Geometry: see drawing. Coordinates: mm, zero at the bounding-box minimum. A direction names the side the tool comes from. Round coordinates to 2 decimals unless told otherwise and drop trailing zeros. Loops run counter-clockwise (first coordinate to the right, second up) from the corner with the lowest first, then second, coordinate; pieces in that order, holes last. Notation, with made-up numbers: M -0.5,24 L 46.5,24 A16 ccw 46.5,47 Z; hole C 80.5,15.25 d2. An arc over 180 degrees is marked long. Answer as a JSON object with one key per item and string values.
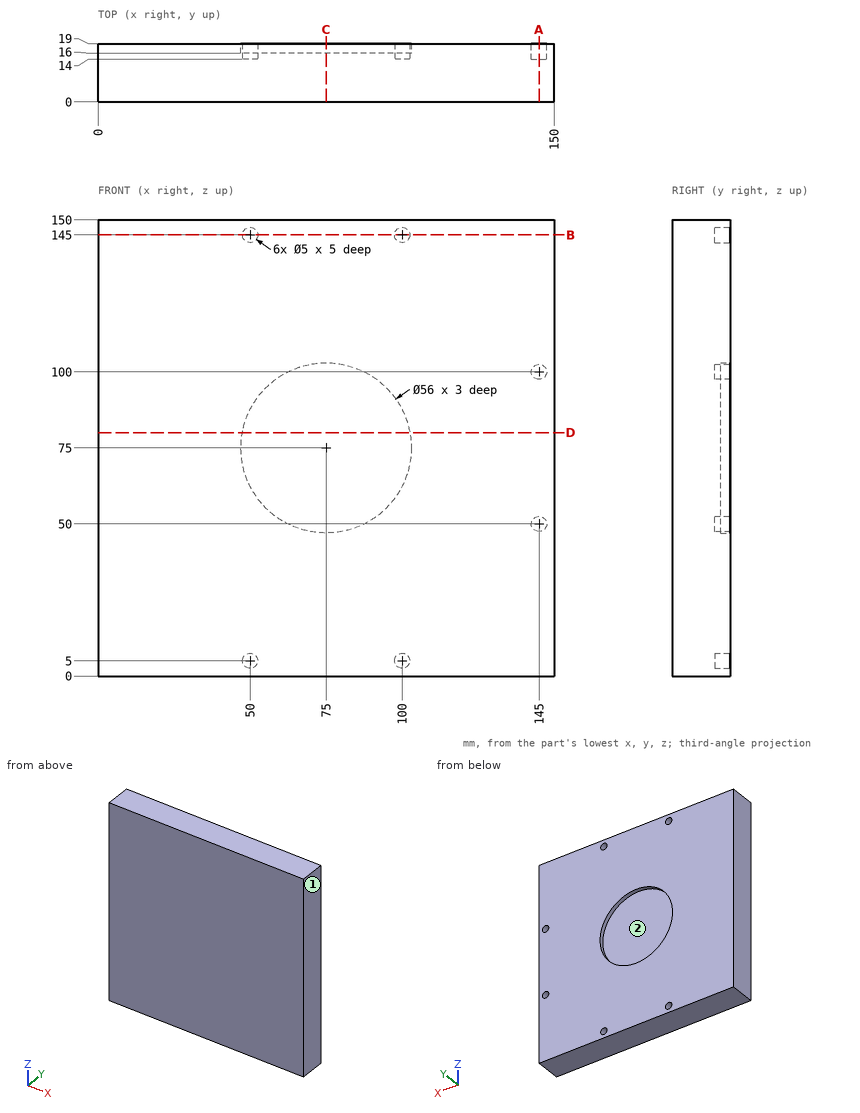
1) Ray query, line 1 (Z direction, x = 145, y = 16.65); line 2 (Z direction, x = 50, y = 15.2). Return the intervals inside material, ascending.
Results:
{"line 1": "0 to 47.5, 52.5 to 97.5, 102.5 to 150", "line 2": "0 to 2.5, 7.5 to 142.5, 147.5 to 150"}
2) Reachability of the marked faces 1 and 2 from +Z, -Z, +X, -X, +Y, -Y: full face, straight path, thin tool, end or side. Return the list, or none.
Results:
{"face 1": "+Z, -Z, +X, +Y, -Y", "face 2": "+Y"}
3) Section query B-B (z = 145). Return the cut outline in (x, y), and give its area (3 significant figures).
Results:
{"outline": "M 0,0 L 150,0 L 150,19 L 102.5,19 L 102.5,14 L 97.5,14 L 97.5,19 L 52.5,19 L 52.5,14 L 47.5,14 L 47.5,19 L 0,19 Z", "area": "2,800 mm2"}
4) Section query D-D (z = 80). Return the cut outline in (x, y).
Results:
{"outline": "M 0,0 L 150,0 L 150,19 L 102.55,19 L 102.55,16 L 47.45,16 L 47.45,19 L 0,19 Z"}
5) Section query C-C (x = 75). Return the cut outline in (y, z).
Results:
{"outline": "M 0,0 L 19,0 L 19,47 L 16,47 L 16,103 L 19,103 L 19,150 L 0,150 Z"}
6) Section query A-A (x = 145). Return the cut outline in (y, z).
Results:
{"outline": "M 0,0 L 19,0 L 19,47.5 L 14,47.5 L 14,52.5 L 19,52.5 L 19,97.5 L 14,97.5 L 14,102.5 L 19,102.5 L 19,150 L 0,150 Z"}
7) Pin query (flat end, axial travel): P1, Ø1.5, axis at x = 145, z = 100.5, coming from the +Y side. Return the tip coordinate at first contact, or that it passes through.
Results:
{"P1": "y = 14"}
